For this review, use the dimensioned drawing (mm, ordinates from the lowest corner) and the shaded views. A direction names the side the tool comes from. Give positions to 0.01 mm unless a question says otherwise; leave off trailing zeros. Write each loop counter-clockwise with the first axis right and the second up, starting at its lowest first coordinate (ties: lowest second). Pieces come first, ordered by that corner, then holes.
1) Wall thickness on line 1 along Y through (x, z) = (3.95, 4.3); line 2 along Z through (x, y) = (2.95, 6.5) (1 decimal); line 3 along X through (y, z) = (7, 2.4) (1 decimal): over which ranges is each line inside the solid? List them lowest first.
2) Machinability: for the marked faces 1 and 2, which of the approach directions +Z, -Z, +X, -X, +Y, -Y give a long, thin tool a straight path to every point of the face, cutting with its end or side? Answer none if there is none.
3) We need section B-B on x = 3.5. Give the boundary of the cut face in (y, z), and give its area (3 significant figures).
4) For P1, Ø1.5, axis at y = 6.5, z = 4.5, coming from the -X side; P2, Ø3, axis at x = 4.5, y = 2, coming from the +Z side; P3, Ø0.8, axis at x = 3, z = 3, coming from the +Y side, all flat-tipped, find the tip position at first contact; note any pin that passes through.
5) Draft analysis for pull direction X (two halves, no side actions). For the marked faces 3, 4 and 5, state which applies: pulls with the +X half, pulls with the -X half, needs draft (parallel to the pull), parting line crosses it, or undercut.
6) We need section C-C on z = 4.7. Give the boundary of the cut face in (x, y).
7) We need section D-D on y = 4. Give the boundary of the cut face in (x, z).
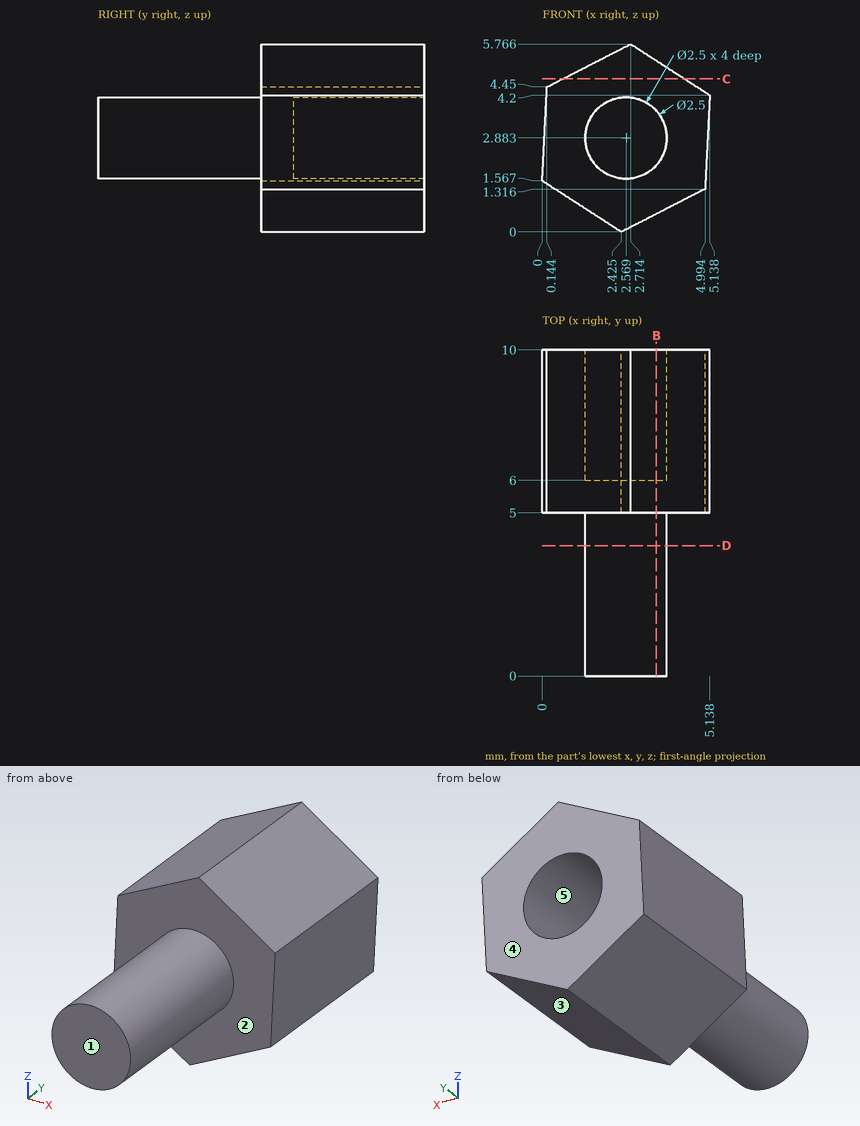
Results list:
1. line 1: y = 5 to 10
1. line 2: z = 0.3 to 1.7, 4.1 to 5.6
1. line 3: x = 0 to 1.4, 3.7 to 5
2. face 1: +Z, -Z, +X, -X, -Y
2. face 2: -Y
3. outline: (0, 2.05) - (5, 2.05) - (5, 0.55) - (10, 0.55) - (10, 2.05) - (6, 2.05) - (6, 3.72) - (10, 3.72) - (10, 5.26) - (5, 5.26) - (5, 3.72) - (0, 3.72) - close
3. area: 25.2 mm2
4. P1: stops at x = 0.11
4. P2: stops at z = 4.06
4. P3: stops at y = 6
5. face 3: pulls with the +X half
5. face 4: needs draft
5. face 5: undercut
6. outline: (0.63, 5) - (4.36, 5) - (4.36, 10) - (0.63, 10) - close
7. outline: circle Ø2.5 at (2.57, 2.88)
